from build123d import *

# Parameters (mm, degrees)
SKETCH1_R           = 4.7371
BOSS_EXTRUDE1_DEPTH = 9.398
SKETCH2_R           = 3.175
BOSS_EXTRUDE2_DEPTH = 78.74
SKETCH3_R           = 4.0259
BOSS_EXTRUDE3_DEPTH = 5.588
SKETCH4_R           = 4.2164
BOSS_EXTRUDE4_DEPTH = 4.5212
SKETCH5_R           = 5.6261
BOSS_EXTRUDE5_DEPTH = 8.2042
SKETCH6_R           = 4.7244
BOSS_EXTRUDE6_DEPTH = 3.81
SKETCH7_R           = 3.1369
BOSS_EXTRUDE7_DEPTH = 3.3528
SKETCH8_R           = 4.7244
BOSS_EXTRUDE8_DEPTH = 7.0866
SKETCH9_R           = 5.3467
BOSS_EXTRUDE9_DEPTH = 18.4658
CHAMFER3_SIZE       = 0.508
CHAMFER3_SIZE2      = 2.54
CHAMFER4_SIZE       = 2.54
CHAMFER4_SIZE2      = 0.680590949
SKETCH10_R          = 2.38125
CUT_EXTRUDE1_DEPTH  = 139.1666


with BuildPart() as part:
    # Sketch1 → Boss-Extrude1 (new body)
    with BuildSketch(Plane.XY):
        Circle(SKETCH1_R)
    extrude(amount=-BOSS_EXTRUDE1_DEPTH)

    # Sketch2 → Boss-Extrude2 (add)
    with BuildSketch(Plane(origin=(0, 0, -9.398), x_dir=(-1, 0, 0), z_dir=(0, 0, -1))):
        Circle(SKETCH2_R)
    extrude(amount=BOSS_EXTRUDE2_DEPTH)

    # Sketch3 → Boss-Extrude3 (add)
    with BuildSketch(Plane(origin=(0, 0, -88.138), x_dir=(-1, 0, 0), z_dir=(0, 0, -1))):
        Circle(SKETCH3_R)
    extrude(amount=BOSS_EXTRUDE3_DEPTH)

    # Sketch4 → Boss-Extrude4 (add)
    with BuildSketch(Plane(origin=(0, 0, -93.726), x_dir=(-1, 0, 0), z_dir=(0, 0, -1))):
        Circle(SKETCH4_R)
    extrude(amount=BOSS_EXTRUDE4_DEPTH)

    # Sketch5 → Boss-Extrude5 (add)
    with BuildSketch(Plane(origin=(0, 0, -98.2472), x_dir=(-1, 0, 0), z_dir=(0, 0, -1))):
        Circle(SKETCH5_R)
    extrude(amount=BOSS_EXTRUDE5_DEPTH)

    # Sketch6 → Boss-Extrude6 (add)
    with BuildSketch(Plane(origin=(0, 0, -106.4514), x_dir=(-1, 0, 0), z_dir=(0, 0, -1))):
        Circle(SKETCH6_R)
    extrude(amount=BOSS_EXTRUDE6_DEPTH)

    # Sketch7 → Boss-Extrude7 (add)
    with BuildSketch(Plane(origin=(0, 0, -110.2614), x_dir=(-1, 0, 0), z_dir=(0, 0, -1))):
        Circle(SKETCH7_R)
    extrude(amount=BOSS_EXTRUDE7_DEPTH)

    # Sketch8 → Boss-Extrude8 (add)
    with BuildSketch(Plane(origin=(0, 0, -113.6142), x_dir=(-1, 0, 0), z_dir=(0, 0, -1))):
        Circle(SKETCH8_R)
    extrude(amount=BOSS_EXTRUDE8_DEPTH)

    # Sketch9 → Boss-Extrude9 (add)
    with BuildSketch(Plane(origin=(0, 0, -120.7008), x_dir=(-1, 0, 0), z_dir=(0, 0, -1))):
        Circle(SKETCH9_R)
    extrude(amount=BOSS_EXTRUDE9_DEPTH)

    # Chamfer3
    chamfer3_edges = [part.edges().sort_by_distance(p)[0] for p in [
        (5.3467, 0, -120.7008),
    ]]
    chamfer3_side = [part.faces().sort_by_distance(p)[0] for p in [
        (5.195472487, 0, -120.7008),
    ]]
    chamfer(chamfer3_edges, length=CHAMFER3_SIZE, length2=CHAMFER3_SIZE2, reference=chamfer3_side[0])

    # Chamfer4
    chamfer4_edges = [part.edges().sort_by_distance(p)[0] for p in [
        (-4.7371, 0, 0),
    ]]
    chamfer4_side = [part.faces().sort_by_distance(p)[0] for p in [
        (-4.7371, 0, -4.699),
    ]]
    chamfer(chamfer4_edges, length=CHAMFER4_SIZE, length2=CHAMFER4_SIZE2, reference=chamfer4_side[0])

    # Sketch10 → Cut-Extrude1 (cut)
    with BuildSketch(Plane.XY):
        Circle(SKETCH10_R)
    extrude(amount=-CUT_EXTRUDE1_DEPTH, mode=Mode.SUBTRACT)


solid = part.part
Part model, mm, in its own coordinate system. A direction names the side the tool comes from. Coordinates: 2 decimals unless noted, no trailing zeros. Write each loop counter-clockwise with the first axis right and the second up, starting at its lowest first coordinate (ties: lowest second). Pieces come first, ordered by that corner, then holes. Notation, with made-up numbers: M -19,60.5 L 30,60.5 A28 ccw 30,85.5 Z; hole C 58,5 d2. An arc over 180 degrees is marked long. Return JSON: item names as keys, results as strings.
1. Probe L1, parallel to Z at x = 2.5, y = -2.25; L2, parallel to Y at x = 0, z = -80 (3 decimals); L3, parallel to Y at x = 0, z = -89.5. List the from-to ranges inside material, lowest first.
Determined:
{"L1": "-139.17 to -113.61, -110.26 to -88.14, -9.4 to 0", "L2": "-3.175 to -2.381, 2.381 to 3.175", "L3": "-4.03 to -2.38, 2.38 to 4.03"}
2. Saw through at A-A, the plane z = -102.5. Write the cut outline in (x, y).
Determined:
{"outline": "C 0,0 d11.25; hole C 0,0 d4.76"}
3. Flat gauge pins, fed straight in: pin 1 Ø1 at (x, z) = (3, -50.5) entering from +Y; pin 2 Ø2.5 at (x, y) = (0, 1) entering from +Z; pin 3 Ø5 at (x, y) = (1, -1.5) entering from +Z; pin 4 Ø3 at (x, z) = (2.5, -106.5) entering from -Y. Where does each tip first touch, or does it go through?
Determined:
{"pin 1": "y = 1.96", "pin 2": "through", "pin 3": "z = 0", "pin 4": "y = -5.54"}
4. Pull direction Z, two halves, no side cores. Call faces 4 (the face through (0.69, -3.1, -48.22)), 5 (the face through (4.243, -3.253, -131.092)), 6 (the face through (-1.1, -2.3, -139.167)): pulls with the +Z half, pulls with the -Z half, needs draft (parallel to the pull), parting line crosses it, or undercut.
Determined:
{"face 4": "undercut", "face 5": "needs draft", "face 6": "pulls with the -Z half"}
5. 3-axis set-ups, long thin cutter, end or side, ignore diameter. For faces 1 (the face through (2, -2, 0)), 2 (the face through (-1.027, -4.624, -5.921)), 3 (the face through (1.1, -3.1, -113.614)): which of +Z, -Z, +X, -X, +Y, -Y reach the whole face in a straight line?
Determined:
{"face 1": "+Z, +X, -X, +Y, -Y", "face 2": "+Z", "face 3": "none"}
